For this review, take the finished solid that the model builds, in its own axes (mm). Round coordinates to 2 decimals unless told otherwise and drop trailing zeros. Loops run counter-clockwise (first coordinate to the right, second up) from the corner with the lowest first, then second, coordinate; pieces in that order, holes last.
1) Take a section at C-C (x = -5.5). State the section outline as (y, z) points.
2) Take a section at D-D (y = -9.5). State the section outline as (x, z) points.
3) Take a section at A-A (y = 33). State the section outline as (x, z) points, then the cut area to 3 significant figures.
4) Take a section at B-B (z = 1). State the section outline as (x, y) points, then the cut area to 3 significant figures.
5) Insertion check: pin 1 (2 mm diameter, centred on x = 24, z = 3.5, fed in from -Y); pin 2 (1 mm diameter, centred on y = -11, z = 4, fed in from -X); pin 3 (1 mm diameter, centred on x = 1, z = 3.5, fed in from -Y). Each pin has a flat end and moves straight along its axis. Give the tip position at first contact, or say it passes through.
6) Wall thickness on L1, parallel to Y at x = 32.5, z = 2.2; L2, parallel to Y at x = 49, z = 2.3; L3, parallel to X at y = 33, z = 0.75: over which ranges is each line inside the solid? List them lowest first.
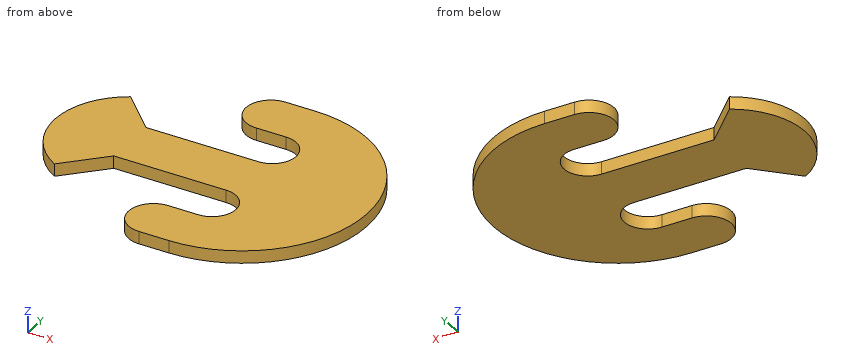
```python
from build123d import *

# Parameters (mm, degrees)
SKETCH1_W           = 45
SKETCH1_H           = 22
BOSS_EXTRUDE1_DEPTH = 5


with BuildPart() as part:
    # Sketch1 → Boss-Extrude1 (new body)
    with BuildSketch(Plane.XY):
        with BuildLine():
            Line((0, 22), (-14.987801249, 36.987801249))
            ThreePointArc((-14.987801249, 36.987801249), (-30, 11), (-14.987801249, -14.987801249))
            Line((-14.987801249, -14.987801249), (0, 0))
            Line((0, 0), (0, 22))
        make_face()
        with Locations((22.5, 11)):
            Rectangle(SKETCH1_W, SKETCH1_H)
        with BuildLine():
            ThreePointArc((45, -19), (54.5, -9.5), (45, 0))
            Line((45, 0), (45, 22))
            ThreePointArc((45, 22), (54.5, 31.5), (45, 41))
            Line((45, 41), (33, 41))
            ThreePointArc((33, 41), (23, 51), (33, 61))
            Line((33, 61), (45, 61))
            ThreePointArc((45, 61), (95, 11), (45, -39))
            Line((45, -39), (33, -39))
            ThreePointArc((33, -39), (23, -29), (33, -19))
            Line((33, -19), (45, -19))
        make_face()
    extrude(amount=BOSS_EXTRUDE1_DEPTH)


solid = part.part
```
Response:
1. outline: (-5.5, 0) - (27.5, 0) - (27.5, 5) - (-5.5, 5) - close
2. outline: (-21.9, 0) - (-9.5, 0) - (-9.5, 5) - (-21.9, 5) - close; (54.5, 0) - (90.6, 0) - (90.6, 5) - (54.5, 5) - close
3. outline: (-20.4, 0) - (-11, 0) - (-11, 5) - (-20.4, 5) - close; (54.38, 0) - (89.9, 0) - (89.9, 5) - (54.38, 5) - close
3. area: 225 mm2
4. outline: (-14.99, -14.99) - (0, 0) - (45, 0) arc R9.5 cw to (45, -19) - (33, -19) arc R10 ccw to (33, -39) - (45, -39) arc R50 ccw to (45, 61) - (33, 61) arc R10 ccw to (33, 41) - (45, 41) arc R9.5 cw to (45, 22) - (0, 22) - (-14.99, 36.99) arc R30 ccw to start
4. area: 6,540 mm2
5. pin 1: stops at y = -35
5. pin 2: stops at x = -20.92
5. pin 3: stops at y = 0
6. L1: y = -38.99 to -19.01, 0 to 22, 41.01 to 60.99
6. L2: y = -38.84 to -18.12, -0.88 to 22.88, 40.12 to 60.84
6. L3: x = -20.4 to -11, 54.38 to 89.9
